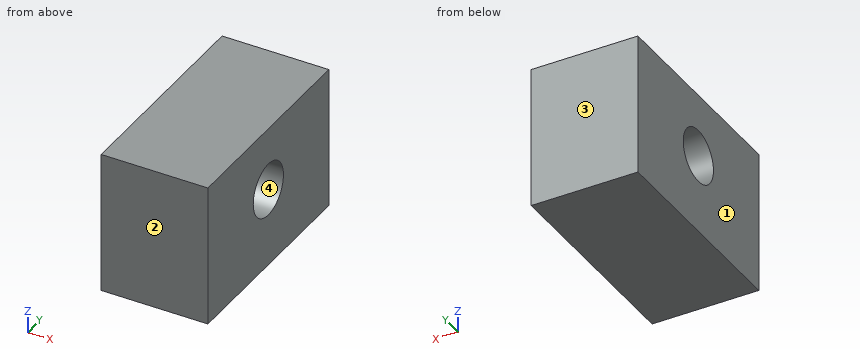
from build123d import *

# Parameters (mm, degrees)
F0_W     = 19.05
F0_H     = 38.1
F1_DEPTH = 25.4
F3_D     = 9.525


with BuildPart() as f1:
    # F0 (on Top) → F1 (new body)
    with BuildSketch(Plane.XY):
        Rectangle(F0_W, F0_H)
    extrude(amount=F1_DEPTH)

    # F3 (through all)
    with Locations(Plane.YZ.offset(9.525)):
        with Locations((0, 14.072823)):
            Hole(F3_D / 2)


solid = f1.part
The model under review builds one solid part; all positions refer to its coordinate system, in mm. Face numbers are marked on the shaded views. Round coordinates to 2 decimals unless told otherwise and drop trailing zeros. Write each loop counter-clockwise with the first axis right and the second up, starting at its lowest first coordinate (ties: lowest second). Pieces come first, ordered by that corner, then holes. Notation, with made-up numbers: (-21, 7.5) - (-10, 7.5) arc R9 ccw to (-10, 19.5) - close; hole circle Ø3 at (23, 11). An arc over 180 degrees is marked (long way). One line per item, written item: value. Start each with the question number.
1. Consider section B-B on z = 10.75. Write out the cut boundary in (x, y) (3 decimals), and give its area (3 significant figures).
2. To check wall thickness, follow L1, parallel to Z at x = 3, y = 0; L2, parallel to Y at x = -6, z = 14; L3, parallel to Z at x = 6, y = 3. State the ranges of each line that lie inside material, in increasing order. Write a range as from..to.
3. Consider section A-A on y = 0. Write out the cut boundary in (x, z) (3 decimals), and give its area (3 significant figures).
4. The part is to be moulded in two halves that separate along Y. For the marked faces 1, 2, 3 and 4, say which applies: released by +Y, released by -Y, zero draft, split by the parting line, or undercut.
Checks:
1. outline: (-9.525, -19.05) - (9.525, -19.05) - (9.525, -3.412) - (-9.525, -3.412) - close; (-9.525, 3.412) - (9.525, 3.412) - (9.525, 19.05) - (-9.525, 19.05) - close
1. area: 596 mm^2
2. L1: z = 0..9.31, 18.84..25.4
2. L2: y = -19.05..-4.76, 4.76..19.05
2. L3: z = 0..10.37, 17.77..25.4
3. outline: (-9.525, 0) - (9.525, 0) - (9.525, 9.31) - (-9.525, 9.31) - close; (-9.525, 18.835) - (9.525, 18.835) - (9.525, 25.4) - (-9.525, 25.4) - close
3. area: 302 mm^2
4. face 1: zero draft
4. face 2: released by -Y
4. face 3: released by +Y
4. face 4: undercut
